Verification items for this drawing (mm, ordinates from the low corner). Give positions to 0.01 mm unless a question says otherwise; leave off trailing zeros. Loops run counter-clockwise (first coordinate to the right, second up) from the corner with the lowest first, then second, coordinate; pieces in that order, holes last. Notation, with made-up numbers: (72, 58) -> (129, 58) arc R23 cw to (129, 83) -> close; hole circle Ø6 at (66, -38). An arc over 180 degrees is marked (long way). Answer as a JSON object with one key per item and string values.
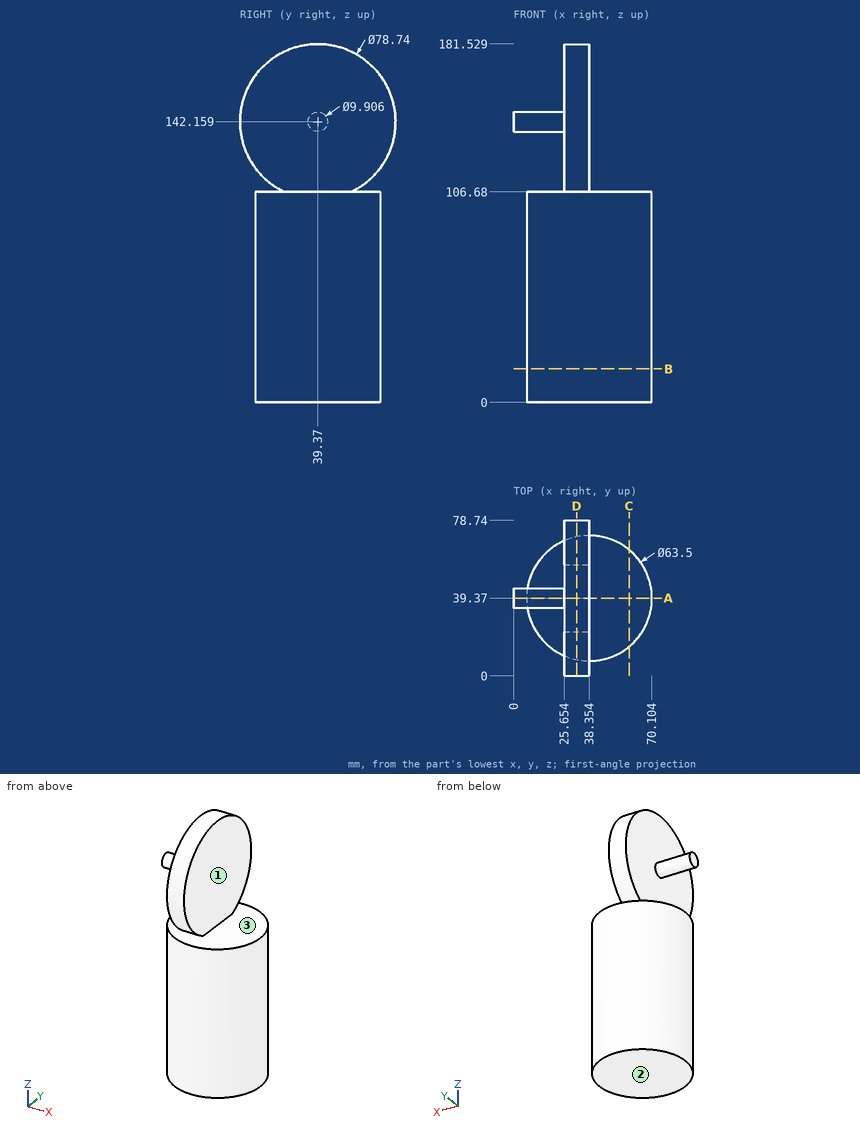
1) Draft check along Z on the marked faces 1, 2 and 3. Enter one of: pulls with the +Z half, pulls with the -Z half, needs draft (parallel to the pull), parting line crosses it, or undercut.
Geometry check:
{"face 1": "needs draft", "face 2": "pulls with the -Z half", "face 3": "undercut"}
2) Section check D-D on x = 32. Record the cut outline in (y, z), plus the area to 3 significant figures.
Geometry check:
{"outline": "(8.26, 0) -> (70.48, 0) -> (70.48, 106.68) -> (56.44, 106.68) arc R39.37 ccw (long way) to (22.3, 106.68) -> (8.26, 106.68) -> close", "area": "11,400 mm2"}
3) Section check C-C on x = 58.5. Record the cut outline in (y, z).
Geometry check:
{"outline": "(14.83, 0) -> (63.91, 0) -> (63.91, 106.68) -> (14.83, 106.68) -> close"}
4) Depth check by flat-ended pin: P1, Ø4, axis at x = 22, z = 67, coming from the +Y side; P2, Ø3, axis at x = 32.5, y = 26.5, coming from the +Z side; P3, Ø2, axis at x = 55.5, y = 31.5, coming from the +Z side. Enter the tip coordinate at first touch or a pass-through.
Geometry check:
{"P1": "stops at y = 67.69", "P2": "stops at z = 179.85", "P3": "stops at z = 106.68"}
5) Section check A-A on y = 39.37. Record the cut outline in (x, z) (1 decimal), plus the area to 3 significant figures.
Geometry check:
{"outline": "(0, 137.2) -> (25.7, 137.2) -> (25.7, 106.7) -> (6.6, 106.7) -> (6.6, 0) -> (70.1, 0) -> (70.1, 106.7) -> (38.4, 106.7) -> (38.4, 181.5) -> (25.7, 181.5) -> (25.7, 147.1) -> (0, 147.1) -> close", "area": "7,980 mm2"}
6) Section check B-B on z = 17. Record the cut outline in (x, y), plus the area to 3 significant figures.
Geometry check:
{"outline": "circle Ø63.5 at (38.35, 39.37)", "area": "3,170 mm2"}
7) Material ranges on line 1 along Z through (x, y) = (49, 24); line 2 along Z through (x, y) = (20.5, 41.5); line 3 along X through (y, z) = (38, 111), recorded low to high. Write a range as from..to.
Geometry check:
{"line 1": "z = 0..106.68", "line 2": "z = 0..106.68, 137.69..146.63", "line 3": "x = 25.65..38.35"}
